Could you check a few things on this drawing? It's one solid part, dimensions in mm from its lowest x, y, z. A direction names the side the tool comes from. Give positions to 0.01 mm unless a question says otherwise; leave off trailing zeros. Order: outer loops, then holes, each group sorted by start corner. A loop starts at its lowest first (then second) coordinate and runs counter-clockwise, first axis right, second up. Notation, with made-up numbers: (41, 1) - (79, 1) arc R26 cw to (79, 29) - close; hole circle Ø5 at (42, -35.75). An arc over 180 degrees is marked (long way). Return JSON: item names as keys, results as strings.
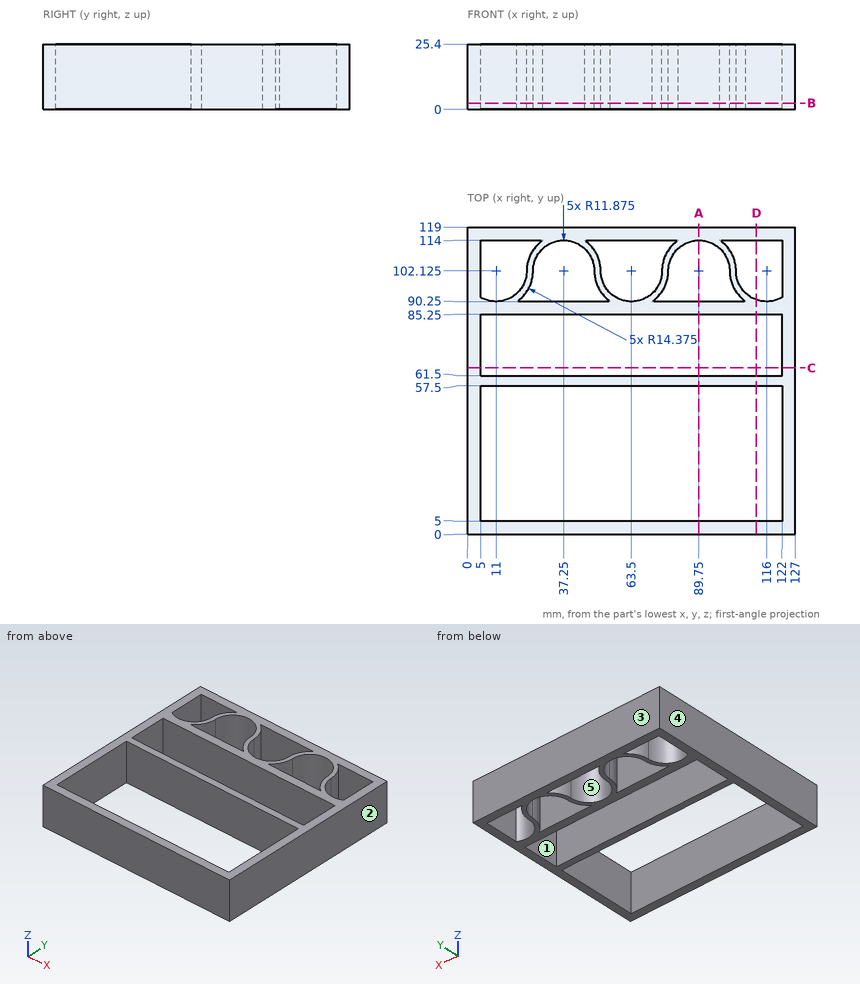
1. Suppose I cut it at D-D (x = 112). List the corners of the cut face in (y, z) for me.
Checks:
{"outline": "(0, 0) - (5, 0) - (5, 25.4) - (0, 25.4) - close; (57.5, 0) - (61.5, 0) - (61.5, 25.4) - (57.5, 25.4) - close; (85.25, 0) - (90.94, 0) - (90.94, 25.4) - (85.25, 25.4) - close; (114, 0) - (119, 0) - (119, 25.4) - (114, 25.4) - close"}
2. Suppose I cut it at C-C (y = 64.5). List the corners of the cut face in (x, z) for me, plus the area to 3 significant figures.
Checks:
{"outline": "(0, 0) - (5, 0) - (5, 25.4) - (0, 25.4) - close; (122, 0) - (127, 0) - (127, 25.4) - (122, 25.4) - close", "area": "254 mm^2"}
3. Suppose I cut it at B-B (z = 2.5). State how many separate pieces and enclosed holes the cut face has, plus the area to 3 significant figures.
Checks:
{"separate pieces": "1", "enclosed holes": "7", "area": "3,720 mm^2"}
4. If I drill on L1, parallel to Y at x = 63.5, z = 23.75; L2, parallel to X at y = 9, z = 11; L3, parallel to Y at x = 74, z = 17.5, over which ranges is the centre line in solid material (lowest first)? Write a range as [from, to].
Checks:
{"L1": "[0, 5], [57.5, 61.5], [85.25, 90.25], [114, 119]", "L2": "[0, 5], [122, 127]", "L3": "[0, 5], [57.5, 61.5], [85.25, 90.25], [92.31, 96.58], [114, 119]"}
5. Suppose I cut it at A-A (x = 89.75). List the corners of the cut face in (y, z) for me.
Checks:
{"outline": "(0, 0) - (5, 0) - (5, 25.4) - (0, 25.4) - close; (57.5, 0) - (61.5, 0) - (61.5, 25.4) - (57.5, 25.4) - close; (85.25, 0) - (90.25, 0) - (90.25, 25.4) - (85.25, 25.4) - close; (114, 0) - (119, 0) - (119, 25.4) - (114, 25.4) - close"}
6. Thinking about a two-plate mould opening in Y: for the marked faces 1, 2 and 3, which applies, +Y half, -Y half, draft (parallel to the pull), parting line (faces both ways), or undercut?
Checks:
{"face 1": "undercut", "face 2": "draft", "face 3": "+Y half"}
7. On a 3-axis mill with a long thin cutter (end or side, diameter ignored), from which of +Z, -Z, +X, -X, +Y, -Y can I reach the whole of each face in a straight line? I mean the marked faces 4 and 5. Say none if no direction works.
Checks:
{"face 4": "+Z, -Z, -X, +Y, -Y", "face 5": "+Z, -Z"}
